Read the model definition and answer for the solid it produces. Units are mm, in the model's axes. A direction names the side the tool comes from. Round coordinates to 2 decimals unless told otherwise and drop trailing zeros. Order: outer loops, then holes, each group sorted by start corner. A loop starts at its lowest first (then second) coordinate and runs counter-clockwise, first axis right, second up.
from build123d import *

# Parameters (mm, degrees)
F0_W         = 47
F0_H         = 47
F1_DEPTH     = 49
F3_DEPTH     = 40
F4_T1_DEPTH  = 37
F4_T3_DEPTH  = 54.5
F4_T5_DEPTH  = 39
F4_T7_DEPTH  = 25
F4_T9_DEPTH  = 47.5
F4_S13_W     = 5
F4_S13_H     = 5
F4_T14_DEPTH = 5
F4_S19_W     = 5
F4_S19_H     = 5
F4_T20_DEPTH = 5
F4_S25_W     = 5
F4_S25_H     = 5
F4_T26_DEPTH = 5
F4_S31_W     = 5
F4_S31_H     = 5
F4_T32_DEPTH = 5
F4_T36_ANGLE = 90
F4_T38_ANGLE = 90
F6_R         = 2.75
F7_DEPTH     = 21
F8_W         = 15
F8_H         = 21
F9_DEPTH     = 4
F10_W        = 3
F10_H        = 6
F10_W_2      = 12
F10_H_2      = 2
F11_DEPTH    = 3.0010001


# Not quite as in the source:
# - a fillet or chamfer that OpenCascade refuses, or shapes differently, is made with other operations: its cross-section is extruded or revolved along the edge and cut away or added


with BuildPart() as f1:
    # F0 (on Front) → F1 (new body)
    with BuildSketch(Plane.XZ):
        with Locations((-31.9517639409, 6.0313746929)):
            Rectangle(F0_W, F0_H)
    extrude(amount=F1_DEPTH)

    # F2 (on face) → F3 (cut)
    with BuildSketch(Plane.YZ.offset(-8.4517639409)):
        with BuildLine():
            Line((-12, 22.5313746929), (-37, 22.5313746929))
            ThreePointArc((-37, 22.5313746929), (-40.5355339059, 21.0669085988), (-42, 17.5313746929))
            Line((-42, 17.5313746929), (-42, -17.4686253071))
            Line((-42, -17.4686253071), (-7, -17.4686253071))
            Line((-7, -17.4686253071), (-7, 17.5313746929))
            ThreePointArc((-7, 17.5313746929), (-8.4644660941, 21.0669085988), (-12, 22.5313746929))
        make_face()
    extrude(amount=-F3_DEPTH, mode=Mode.SUBTRACT)

    # F4: fillet of radius 5 on 9 edges, made by hand

    # F4_s2 → F4_t1 (cut)
    with BuildSketch(Plane.YZ.offset(-50.4517639409)):
        with BuildLine():
            ThreePointArc((-44, 29.5313746929), (-47.5355339059, 28.0669085988), (-49, 24.5313746929))
            Line((-49, 24.5313746929), (-49, 29.5313746929))
            Line((-49, 29.5313746929), (-44, 29.5313746929))
        make_face()
        with BuildLine():
            ThreePointArc((0, 24.5313746929), (-1.4644660941, 28.0669085988), (-5, 29.5313746929))
            Line((-5, 29.5313746929), (0, 29.5313746929))
            Line((0, 29.5313746929), (0, 24.5313746929))
        make_face()
    extrude(amount=F4_T1_DEPTH, mode=Mode.SUBTRACT)

    # F4_s4 → F4_t3 (cut)
    with BuildSketch(Plane.XY.offset(-29.9686253071)):
        with BuildLine():
            ThreePointArc((-8.4517639409, -44), (-9.9162300349, -47.5355339059), (-13.4517639409, -49))
            Line((-13.4517639409, -49), (-8.4517639409, -49))
            Line((-8.4517639409, -49), (-8.4517639409, -44))
        make_face()
        with BuildLine():
            ThreePointArc((-8.4517639409, -5), (-9.9162300349, -1.4644660941), (-13.4517639409, 0))
            Line((-13.4517639409, 0), (-8.4517639409, 0))
            Line((-8.4517639409, 0), (-8.4517639409, -5))
        make_face()
        with BuildLine():
            ThreePointArc((-50.4517639409, 0), (-53.9872978468, -1.4644660941), (-55.4517639409, -5))
            Line((-55.4517639409, -5), (-55.4517639409, 0))
            Line((-55.4517639409, 0), (-50.4517639409, 0))
        make_face()
        with BuildLine():
            ThreePointArc((-50.4517639409, -49), (-53.9872978468, -47.5355339059), (-55.4517639409, -44))
            Line((-55.4517639409, -44), (-55.4517639409, -49))
            Line((-55.4517639409, -49), (-50.4517639409, -49))
        make_face()
    extrude(amount=F4_T3_DEPTH, mode=Mode.SUBTRACT)

    # F4_s6 → F4_t5 (cut)
    with BuildSketch(Plane.XZ.offset(5)):
        with BuildLine():
            ThreePointArc((-8.4517639409, 24.5313746929), (-9.9162300349, 28.0669085988), (-13.4517639409, 29.5313746929))
            Line((-13.4517639409, 29.5313746929), (-8.4517639409, 29.5313746929))
            Line((-8.4517639409, 29.5313746929), (-8.4517639409, 24.5313746929))
        make_face()
        with BuildLine():
            ThreePointArc((-50.4517639409, 29.5313746929), (-53.9872978468, 28.0669085988), (-55.4517639409, 24.5313746929))
            Line((-55.4517639409, 24.5313746929), (-55.4517639409, 29.5313746929))
            Line((-55.4517639409, 29.5313746929), (-50.4517639409, 29.5313746929))
        make_face()
    extrude(amount=F4_T5_DEPTH, mode=Mode.SUBTRACT)

    # F4_s8 → F4_t7 (cut)
    with BuildSketch(Plane.XZ.offset(12)):
        with BuildLine():
            ThreePointArc((-8.4517639409, 27.5313746929), (-9.9162300349, 23.995840787), (-13.4517639409, 22.5313746929))
            Line((-13.4517639409, 22.5313746929), (-8.4517639409, 22.5313746929))
            Line((-8.4517639409, 22.5313746929), (-8.4517639409, 27.5313746929))
        make_face()
    extrude(amount=F4_T7_DEPTH, mode=Mode.SUBTRACT)

    # F4_s10 → F4_t9 (cut)
    with BuildSketch(Plane.XY.offset(-29.9686253071)):
        with BuildLine():
            ThreePointArc((-8.4517639409, -47), (-9.9162300349, -43.4644660941), (-13.4517639409, -42))
            Line((-13.4517639409, -42), (-8.4517639409, -42))
            Line((-8.4517639409, -42), (-8.4517639409, -47))
        make_face()
        with BuildLine():
            ThreePointArc((-8.4517639409, -2), (-9.9162300349, -5.5355339059), (-13.4517639409, -7))
            Line((-13.4517639409, -7), (-8.4517639409, -7))
            Line((-8.4517639409, -7), (-8.4517639409, -2))
        make_face()
    extrude(amount=F4_T9_DEPTH, mode=Mode.SUBTRACT)


with BuildPart() as f4_tool12:
    # F4_s13 → F4_t14 (new body)
    with BuildSketch(Plane.YZ.offset(-13.4517639409)):
        with Locations((-46.5, 27.0313746929)):
            Rectangle(F4_S13_W, F4_S13_H)
    extrude(amount=F4_T14_DEPTH)

    # F4_s15 → F4_t16 (revolve, cut)
    with BuildSketch(Plane(origin=(-13.4517639409, -44, 24.5313746929), x_dir=(0, 0.7071067812, -0.7071067812), z_dir=(0, -0.7071067812, -0.7071067812))):
        with BuildLine():
            ThreePointArc((0, -5), (5, 0), (0, 5))
            Line((0, 5), (0, -5))
        make_face()
    revolve(axis=Axis((-13.4517639409, -44, 24.5313746929), (1, 0, 0)), mode=Mode.SUBTRACT)


with BuildPart() as f1_1:
    add(f1.part)

    # F4_t11: cut F4_tool12
    add(f4_tool12.part, mode=Mode.SUBTRACT)


with BuildPart() as f4_tool18:
    # F4_s19 → F4_t20 (new body)
    with BuildSketch(Plane.YZ.offset(-50.4517639409)):
        with Locations((-46.5, 27.0313746929)):
            Rectangle(F4_S19_W, F4_S19_H)
    extrude(amount=-F4_T20_DEPTH)

    # F4_s21 → F4_t22 (revolve, cut)
    with BuildSketch(Plane(origin=(-50.4517639409, -44, 24.5313746929), x_dir=(0, 0.7071067812, -0.7071067812), z_dir=(0, 0.7071067812, 0.7071067812))):
        with BuildLine():
            ThreePointArc((0, -5), (5, 0), (0, 5))
            Line((0, 5), (0, -5))
        make_face()
    revolve(axis=Axis((-50.4517639409, -44, 24.5313746929), (-1, 0, 0)), mode=Mode.SUBTRACT)


with BuildPart() as f1_2:
    add(f1_1.part)

    # F4_t17: cut F4_tool18
    add(f4_tool18.part, mode=Mode.SUBTRACT)


with BuildPart() as f4_tool24:
    # F4_s25 → F4_t26 (new body)
    with BuildSketch(Plane.YZ.offset(-13.4517639409)):
        with Locations((-2.5, 27.0313746929)):
            Rectangle(F4_S25_W, F4_S25_H)
    extrude(amount=F4_T26_DEPTH)

    # F4_s27 → F4_t28 (revolve, cut)
    with BuildSketch(Plane(origin=(-13.4517639409, -5, 24.5313746929), x_dir=(0, -0.7071067812, -0.7071067812), z_dir=(0, -0.7071067812, 0.7071067812))):
        with BuildLine():
            ThreePointArc((0, -5), (5, 0), (0, 5))
            Line((0, 5), (0, -5))
        make_face()
    revolve(axis=Axis((-13.4517639409, -5, 24.5313746929), (1, 0, 0)), mode=Mode.SUBTRACT)


with BuildPart() as f1_3:
    add(f1_2.part)

    # F4_t23: cut F4_tool24
    add(f4_tool24.part, mode=Mode.SUBTRACT)


with BuildPart() as f4_tool30:
    # F4_s31 → F4_t32 (new body)
    with BuildSketch(Plane.XZ.offset(5)):
        with Locations((-52.9517639409, 27.0313746929)):
            Rectangle(F4_S31_W, F4_S31_H)
    extrude(amount=-F4_T32_DEPTH)

    # F4_s33 → F4_t34 (revolve, cut)
    with BuildSketch(Plane(origin=(-50.4517639409, -5, 24.5313746929), x_dir=(0.7071067812, 0, -0.7071067812), z_dir=(0.7071067812, 0, 0.7071067812))):
        with BuildLine():
            ThreePointArc((0, -5), (5, 0), (0, 5))
            Line((0, 5), (0, -5))
        make_face()
    revolve(axis=Axis((-50.4517639409, -5, 24.5313746929), (0, 1, 0)), mode=Mode.SUBTRACT)


with BuildPart() as f1_4:
    add(f1_3.part)

    # F4_t29: cut F4_tool30
    add(f4_tool30.part, mode=Mode.SUBTRACT)

    # F4_s35 → F4_t36 (revolve, cut)
    with BuildSketch(Plane.XY.offset(17.5313746929)):
        with BuildLine():
            ThreePointArc((-8.4517639409, -2), (-9.9162300349, -5.5355339059), (-13.4517639409, -7))
            Line((-13.4517639409, -7), (-8.4517639409, -7))
            Line((-8.4517639409, -7), (-8.4517639409, -2))
        make_face()
    revolve(axis=Axis((-8.4517639409, -12, 17.5313746929), (1, 0, 0)), revolution_arc=F4_T36_ANGLE, mode=Mode.SUBTRACT)

    # F4_s37 → F4_t38 (revolve, cut)
    with BuildSketch(Plane.XZ.offset(37)):
        with BuildLine():
            ThreePointArc((-8.4517639409, 27.5313746929), (-9.9162300349, 23.995840787), (-13.4517639409, 22.5313746929))
            Line((-13.4517639409, 22.5313746929), (-8.4517639409, 22.5313746929))
            Line((-8.4517639409, 22.5313746929), (-8.4517639409, 27.5313746929))
        make_face()
    revolve(axis=Axis((-8.4517639409, -37, 17.5313746929), (1, 0, 0)), revolution_arc=F4_T38_ANGLE, mode=Mode.SUBTRACT)

    # F6 (on offset) → F7 (cut)
    with BuildSketch(Plane.XZ.offset(14.5)):
        with Locations((-45.4517639409, 24.5701503009)):
            Circle(F6_R)
    extrude(amount=F7_DEPTH, mode=Mode.SUBTRACT)

    # F8 (on face) → F9 (cut)
    with BuildSketch(Plane(origin=(0, 0, 22.5313746929), x_dir=(1, 0, 0), z_dir=(0, 0, -1))):
        with Locations((-34.8641358682, 25)):
            Rectangle(F8_W, F8_H)
    extrude(amount=-F9_DEPTH, mode=Mode.SUBTRACT)

    # F10 (on face) → F11 (cut, through all)
    with BuildSketch(Plane(origin=(0, 0, 26.5313746929), x_dir=(1, 0, 0), z_dir=(0, 0, -1))):
        with Locations((-28.8641358682, 30.5)):
            Rectangle(F10_W, F10_H)
        Polygon((-30.3641358682, 22.5), (-30.3641358682, 16.5), (-30.3641358682, 14.5), (-27.3641358682, 14.5), (-27.3641358682, 22.5), align=None)
        with Locations((-36.3641358682, 34.5)):
            Rectangle(F10_W_2, F10_H_2)
        with Locations((-28.8641358682, 34.5)):
            Rectangle(F10_W, F10_H_2)
        with Locations((-36.3641358682, 15.5)):
            Rectangle(F10_W_2, F10_H_2)
    extrude(amount=-F11_DEPTH, mode=Mode.SUBTRACT)


solid = f1_4.part
Q1. A cutting plane is placed at C-C, the plane z = -9. Give the vertices of the cut face in (x, y), plus the area to 3 significant figures.
Outcome:
outline: (-55.45, -44) arc R5 ccw to (-50.45, -49) - (-13.45, -49) arc R5 ccw to (-8.68, -45.5) arc R5 ccw to (-13.45, -42) - (-48.45, -42) - (-48.45, -7) - (-13.45, -7) arc R5 ccw to (-8.68, -3.5) arc R5 ccw to (-13.45, 0) - (-50.45, 0) arc R5 ccw to (-55.45, -5) - close
area: 871 mm2
Q2. A cutting plane is placed at D-D, the plane y = -13. Give the vertices of the cut face in (x, z).
Outcome:
outline: (-55.45, -17.47) - (-48.45, -17.47) - (-48.45, 22.53) - (-13.45, 22.53) arc R5 ccw to (-8.68, 26.03) arc R5 ccw to (-13.45, 29.53) - (-50.45, 29.53) arc R5 ccw to (-55.45, 24.53) - close
Q3. For faces 1 (the face through (-10.458, -24.325, 23.527)), 2 (the face through (-32.2, -1.4, 28)), 3 (the face through (-32.2, -47.5, 28.1)), 4 (the face through (-45, -14.5, 25)), 5 (the face through (-30.364, -20, 28)), determine the directions among +Z, -Z, +X, -X, +Y, -Y from which every point of the face is accessible in a straight line to the end or side of a thin tool.
Outcome:
face 1: -Z, +X
face 2: +Z, +X, -X, +Y
face 3: +Z, +X, -X, -Y
face 4: none
face 5: +Z, -Z
Q4. Straight lines are drawn through the part: probe 1 along Y at (x, z) = (-41, 16.5); probe 2 along X at (y, z) = (-21.5, 21); probe 3 along Z at (x, y) = (-19.5, -25.5). For each, find the intervals that lie inside material, in ascending order.
Outcome:
probe 1: y = -49 to -42, -7 to 0
probe 2: x = -55.45 to -48.45
probe 3: z = 22.53 to 29.53
Q5. A cutting plane is placed at B-B, the plane y = -31. Give the vertices of the cut face in (x, z), plus the area to 3 significant figures.
Outcome:
outline: (-55.45, -17.47) - (-48.45, -17.47) - (-48.45, 22.53) - (-47.3, 22.53) arc R2.75 cw (long way) to (-43.61, 22.53) - (-42.36, 22.53) - (-42.36, 26.53) - (-30.36, 26.53) - (-30.36, 29.53) - (-50.45, 29.53) arc R5 ccw to (-55.45, 24.53) - close; (-27.36, 22.53) - (-13.45, 22.53) arc R5 ccw to (-8.68, 26.03) arc R5 ccw to (-13.45, 29.53) - (-27.36, 29.53) - close
area: 502 mm2
Q6. For a pull along Z with two mould halves and no side action, classify faces 6 (the face through (-45.36, -24.85, 27.32)), 7 (the face through (-30.7, -8.4, 21)), 8 (the face through (-10.458, -6.005, -0.214)) as released by +Z, released by -Z, zero draft, split by the parting line, or undercut.
Outcome:
face 6: undercut
face 7: released by -Z
face 8: zero draft
Q7. A cutting plane is placed at A-A, the plane x = -35.5. Give the vertices of the cut face in (y, z).
Outcome:
outline: (-49, -17.47) - (-42, -17.47) - (-42, 17.53) arc R5 cw to (-37, 22.53) - (-35.5, 22.53) - (-35.5, 29.53) - (-44, 29.53) arc R5 ccw to (-49, 24.53) - close; (-33.5, 26.53) - (-16.5, 26.53) - (-16.5, 29.53) - (-33.5, 29.53) - close; (-14.5, 22.53) - (-12, 22.53) arc R5 cw to (-7, 17.53) - (-7, -17.47) - (0, -17.47) - (0, 24.53) arc R5 ccw to (-5, 29.53) - (-14.5, 29.53) - close
Q8. Flat-ended cylindrical pins translate along their axes: pin 1 (1.5 mm diameter, centred on y = -19, z = 28.5, fed in from +X); pin 2 (3.5 mm diameter, centred on x = -34.5, z = 28.5, fed in from +Y); pin 3 (2.5 mm diameter, centred on x = -29.5, z = 28.5, fed in from +Y). Find the tip coordinate at first contact, or state that the pin passes through.
Outcome:
pin 1: stops at x = -9.63
pin 2: stops at y = -0.52
pin 3: stops at y = -0.8
